Model file for the job. Use its own axes, mm. Face numbers are marked on the shaded views. A direction names the side the tool comes from. Round coordinates to 2 decimals unless told otherwise and drop trailing zeros. Order: outer loops, then holes, each group sorted by start corner. A loop starts at its lowest first (then second) coordinate and runs counter-clockwise, first axis right, second up. Notation, with made-up numbers: M 56,54 L 64,54 A36 cw 64,91 Z; hole C -12.75,17 d11. An arc over 180 degrees is marked long. Return JSON: item names as keys, results as strings. Group by question number.
Item 1: Pin check, flat tip, straight feed: pin 1 Ø6 at (x, z) = (163.5, -143.5) entering from +Y. Stop position of the tip, or through.
Item 2: Slice it at A-A on x = 279.4. Write the cut outline in (y, z).
Item 3: Slice it at D-D on z = -57.5. Write the cut outline in (x, y), then the cut area to 3 significant figures.
Item 4: Slice it at C-C on y = 62.5. Write the cut outline in (x, z).
Item 5: Which spindle directions (+Z, -Z, +X, -X, +Y, -Y) get a long thin tool onto all of the face, cutting with end or side? Do the marked faces 1 and 2. Say none if no direction does.
Item 6: Probe line 1 along Y through (x, z) = (279.4, 12.25); line 2 along Y through (x, z) = (62, -55.5); line 3 along Y through (x, z) = (139.7, 11.75). List the from-to ranges inside material, lowest first.
Item 7: Slice it at B-B on x = 139.7. Write the cut outline in (y, z), then the cut area to 3 significant figures.
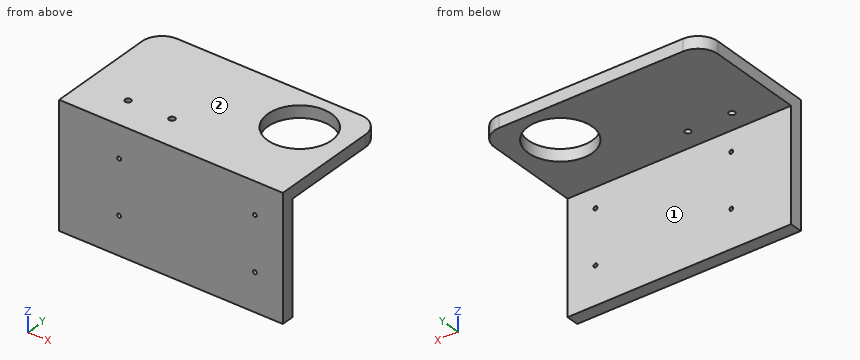
from build123d import *

# Parameters (mm, degrees)
SKETCH1_W           = 355.6
SKETCH1_H           = 177.8
SKETCH1_R           = 3.048
BOSS_EXTRUDE1_DEPTH = 19.939
SKETCH2_W           = 355.6
SKETCH2_H           = 19.05
BOSS_EXTRUDE2_DEPTH = 203.2
SKETCH3_R           = 50.8
SKETCH3_R_2         = 4.7625
CUT_EXTRUDE1_DEPTH  = 455.413382835
FILLET1_R           = 31.75


with BuildPart() as part:
    # Sketch1 → Boss-Extrude1 (new body)
    with BuildSketch(Plane(origin=(0, 0, 0), x_dir=(1, 0, 0), z_dir=(0, 1, 0))):
        with Locations((177.8, 88.9)):
            Rectangle(SKETCH1_W, SKETCH1_H)
        with Locations(Location((95.25, 117.475, 0), (0, 0, 270))):
            Circle(SKETCH1_R, mode=Mode.SUBTRACT)
        with Locations(Location((311.15, 117.475, 0), (0, 0, 270))):
            Circle(SKETCH1_R, mode=Mode.SUBTRACT)
        with Locations(Location((311.15, 31.75, 0), (0, 0, 270))):
            Circle(SKETCH1_R, mode=Mode.SUBTRACT)
        with Locations(Location((95.25, 31.75, 0), (0, 0, 270))):
            Circle(SKETCH1_R, mode=Mode.SUBTRACT)
    extrude(amount=BOSS_EXTRUDE1_DEPTH)

    # Sketch2 → Boss-Extrude2 (add)
    with BuildSketch(Plane(origin=(0, 0, 0), x_dir=(1, 0, 0), z_dir=(0, 1, 0))):
        with Locations((177.8, -9.525)):
            Rectangle(SKETCH2_W, SKETCH2_H)
    extrude(amount=BOSS_EXTRUDE2_DEPTH)

    # Sketch3 → Cut-Extrude1 (cut, through all)
    with BuildSketch(Plane.XY.offset(19.05)):
        with Locations((279.4, 134.239)):
            Circle(SKETCH3_R)
        with Locations((69.85, 51.689)):
            Circle(SKETCH3_R_2)
        with Locations((139.7, 51.689)):
            Circle(SKETCH3_R_2)
    extrude(amount=-CUT_EXTRUDE1_DEPTH, mode=Mode.SUBTRACT)

    # Fillet1
    fillet1_edges = [part.edges().sort_by_distance(p)[0] for p in [
        (355.6, 203.2, 9.525),
        (0, 203.2, 9.525),
    ]]
    fillet(fillet1_edges, radius=FILLET1_R)


solid = part.part
Output values:
{
 "1": {"pin 1": "y = 19.94"},
 "2": {"outline": "M 0,-177.8 L 19.94,-177.8 L 19.94,0 L 83.44,0 L 83.44,19.05 L 0,19.05 Z; M 185.04,0 L 203.2,0 L 203.2,19.05 L 185.04,19.05 Z"},
 "3": {"outline": "M 0,0 L 355.6,0 L 355.6,19.94 L 0,19.94 Z", "area": "7,090 mm²"},
 "4": {"outline": "M 0,0 L 355.6,0 L 355.6,19.05 L 0,19.05 Z"},
 "5": {"face 1": "-Z, +X, -X, +Y", "face 2": "+Z, +X, -X, +Y, -Y"},
 "6": {"line 1": "0 to 83.44, 185.04 to 203.2", "line 2": "0 to 19.94", "line 3": "0 to 46.93, 56.45 to 203.2"},
 "7": {"outline": "M 0,-177.8 L 19.94,-177.8 L 19.94,0 L 46.93,0 L 46.93,19.05 L 0,19.05 Z; M 56.45,0 L 203.2,0 L 203.2,19.05 L 56.45,19.05 Z", "area": "7,230 mm²"}
}
